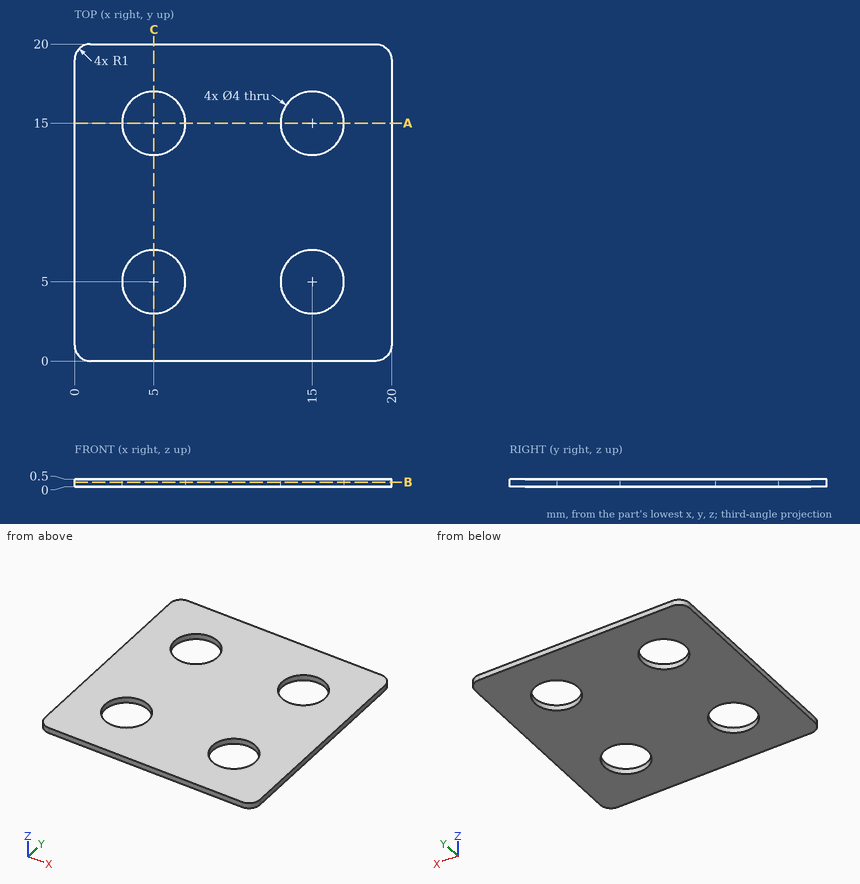
The drawing under review shows one solid part. Ordinate dimensions are in mm from its lowest x, y, z. Coordinates: 2 decimals unless noted, no trailing zeros. Loops run counter-clockwise (first coordinate to the right, second up) from the corner with the lowest first, then second, coordinate; pieces in that order, holes last. Notation, with made-up numbers: (2, 80) - (24, 80) arc R20 ccw to (24, 97) - close; hole circle Ø11 at (2, 70). An arc over 180 degrees is marked (long way). Return JSON: item names as keys, results as strings.
Item 1: For line 1 (Y direction, x = 15, z = 0.35); line 2 (X direction, y = 15.75, z = 0.4); line 3 (Y direction, x = 6.5, z = 0.1), list the stretches that pass through material, from the lowest coordinate up.
Determined:
{"line 1": "y = 0 to 3, 7 to 13, 17 to 20", "line 2": "x = 0 to 3.15, 6.85 to 13.15, 16.85 to 20", "line 3": "y = 0 to 3.68, 6.32 to 13.68, 16.32 to 20"}
Item 2: Take a section at B-B (z = 0.3). Give the boundary of the cut face in (x, y).
Determined:
{"outline": "(0, 1) arc R1 ccw to (1, 0) - (19, 0) arc R1 ccw to (20, 1) - (20, 19) arc R1 ccw to (19, 20) - (1, 20) arc R1 ccw to (0, 19) - close; hole circle Ø4 at (5, 5); hole circle Ø4 at (5, 15); hole circle Ø4 at (15, 5); hole circle Ø4 at (15, 15)"}
Item 3: Insertion check: pin 1 (3 mm diameter, centred on x = 15, y = 5, fed in from +Z). The pin has a flat end and moves straight along its axis. Give the tip position at first contact, or say it passes through.
Determined:
{"pin 1": "passes through"}
Item 4: Take a section at A-A (y = 15). Give the boundary of the cut face in (x, z).
Determined:
{"outline": "(0, 0) - (3, 0) - (3, 0.5) - (0, 0.5) - close; (7, 0) - (13, 0) - (13, 0.5) - (7, 0.5) - close; (17, 0) - (20, 0) - (20, 0.5) - (17, 0.5) - close"}
